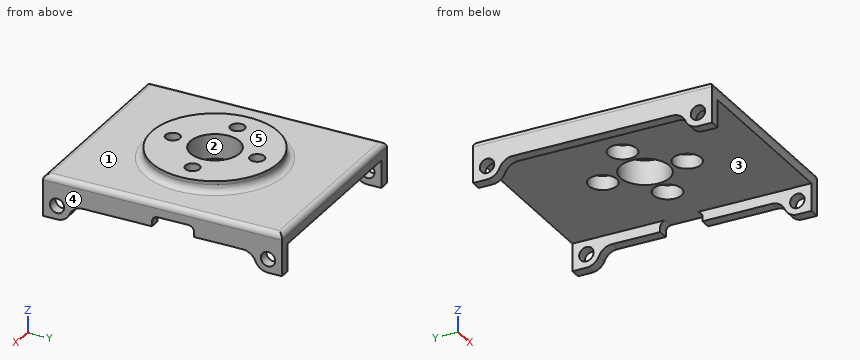
```python
from build123d import *

# Parameters (mm, degrees)
BOSS_EXTRUDE1_DEPTH = 17
SKETCH2_R           = 1.025
CUT_EXTRUDE1_DEPTH  = 50
CUT_EXTRUDE2_DEPTH  = 50
FILLET1_R           = 2
SKETCH8_W           = 1.5
SKETCH8_H           = 6
CUT_EXTRUDE5_DEPTH  = 10
SKETCH9_R           = 9
BOSS_EXTRUDE2_DEPTH = 1.5
SKETCH7_R           = 3.5
SKETCH7_R_2         = 1.025
CUT_EXTRUDE6_DEPTH  = 10
SKETCH10_R          = 2
CUT_EXTRUDE7_DEPTH  = 2
FILLET2_R           = 1
FILLET3_R           = 0.8
FILLET4_R           = 0.8


with BuildPart() as part:
    # Sketch1 → Boss-Extrude1 (new body, symmetric)
    with BuildSketch(Plane(origin=(0, 0, 0), x_dir=(1, 0, 0), z_dir=(0, 1, 0))):
        Polygon((-14, 0), (14, 0), (14, 5.93), (12.5, 5.93), (12.5, 2), (-12.5, 2), (-12.5, 5.93), (-14, 5.93), align=None)
    extrude(amount=BOSS_EXTRUDE1_DEPTH, both=True)

    # Sketch2 → Cut-Extrude1 (cut, symmetric)
    with BuildSketch(Plane(origin=(-12.5, 0, 0), x_dir=(0, 0, -1), z_dir=(1, 0, 0))):
        with Locations((4, 15)):
            Circle(SKETCH2_R)
        with Locations((4, -15)):
            Circle(SKETCH2_R)
    extrude(amount=CUT_EXTRUDE1_DEPTH, both=True, mode=Mode.SUBTRACT)

    # Sketch3 → Cut-Extrude2 (cut, symmetric)
    with BuildSketch(Plane(origin=(14, 0, 0), x_dir=(0, 0, -1), z_dir=(1, 0, 0))):
        with BuildLine():
            Line((3.5, -13.135891634), (3.5, 13.135891634))
            ThreePointArc((3.5, 13.135891634), (5.174712731, 13.468677043), (5.93, 15))
            Line((5.93, 15), (5.93, -15))
            ThreePointArc((5.93, -15), (5.174712731, -13.468677043), (3.5, -13.135891634))
        make_face()
    extrude(amount=CUT_EXTRUDE2_DEPTH, both=True, mode=Mode.SUBTRACT)

    # Fillet1
    fillet1_edges = [part.edges().sort_by_distance(p)[0] for p in [
        (13.25, 13.135891634, -3.5),
        (-13.25, 13.135891634, -3.5),
        (13.25, -13.135891634, -3.5),
        (-13.25, -13.135891634, -3.5),
    ]]
    fillet(fillet1_edges, radius=FILLET1_R)

    # Sketch8 → Cut-Extrude5 (cut)
    with BuildSketch(Plane(origin=(14, 0, 0), x_dir=(0, 0, -1), z_dir=(1, 0, 0))):
        with Locations((2.75, 1.5)):
            Rectangle(SKETCH8_W, SKETCH8_H)
    extrude(amount=-CUT_EXTRUDE5_DEPTH, mode=Mode.SUBTRACT)

    # Sketch9 → Boss-Extrude2 (add)
    with BuildSketch(Plane.XY):
        Circle(SKETCH9_R)
    extrude(amount=BOSS_EXTRUDE2_DEPTH)

    # Sketch7 → Cut-Extrude6 (cut)
    with BuildSketch(Plane.XY.offset(-2)):
        Circle(SKETCH7_R)
        with Locations((0, 6)):
            Circle(SKETCH7_R_2)
        with Locations((0, -6)):
            Circle(SKETCH7_R_2)
        with Locations((6, 0)):
            Circle(SKETCH7_R_2)
        with Locations((-6, 0)):
            Circle(SKETCH7_R_2)
    extrude(amount=CUT_EXTRUDE6_DEPTH, mode=Mode.SUBTRACT)

    # Sketch10 → Cut-Extrude7 (cut)
    with BuildSketch(Plane(origin=(0, 0, -2), x_dir=(-1, 0, 0), z_dir=(0, 0, -1))):
        with Locations((0, 6)):
            Circle(SKETCH10_R)
        with Locations((-6, 0)):
            Circle(SKETCH10_R)
        with Locations((0, -6)):
            Circle(SKETCH10_R)
        with Locations((6, 0)):
            Circle(SKETCH10_R)
    extrude(amount=-CUT_EXTRUDE7_DEPTH, mode=Mode.SUBTRACT)

    # Fillet2
    fillet2_edges = [part.edges().sort_by_distance(p)[0] for p in [
        (-9, 0, 0),
    ]]
    fillet(fillet2_edges, radius=FILLET2_R)

    # Fillet3
    fillet3_edges = [part.edges().sort_by_distance(p)[0] for p in [
        (14, 0, 0),
        (-14, 0, 0),
        (0, 17, 0),
        (0, -17, 0),
    ]]
    fillet(fillet3_edges, radius=FILLET3_R)

    # Fillet4
    fillet4_edges = [part.edges().sort_by_distance(p)[0] for p in [
        (13.25, -1.5, -2),
        (13.25, 4.5, -2),
    ]]
    fillet(fillet4_edges, radius=FILLET4_R)


solid = part.part
```
Geometry: final body of the model. Coordinates: model frame, mm. Face numbers are marked on the shaded views. A direction names the side the tool comes from. Round coordinates to 2 decimals unless told otherwise and drop trailing zeros. Order: outer loops, then holes, each group sorted by start corner. A loop starts at its lowest first (then second) coordinate and runs counter-clockwise, first axis right, second up. Notation, with made-up numbers: (21.5, -28.5) -> (65.5, -28.5) arc R10 cw to (65.5, -20.5) -> close; hole circle Ø9 at (24.5, 61). An arc over 180 degrees is marked (long way). Use CSV: the item, a comma, the result in double quotes. Start each with the question number.
1) Set-up query: the marked faces 1 and 2. Return all of +Z, -Z, +X, -X, +Y, -Y with unobstructed straight access to the full face (end or side cutting, diameter ignored); none if empty.
2) Section A-A (y = 0). State how many separate pieces and enclosed holes the cut face has, and give its area (3 significant figures).
3) Material intervals for line 1 along X through (y, z) = (10, -2.5); line 2 along Y through (x, z) = (0, -0.55); line 3 along Y through (x, z) = (13.75, -4) (3 decimals), sorted ascending. Write a range as from..to.
4) Draft query along X for the marked faces 3, 4 and 5. Return one class per face: +X half, -X half, draft (parallel to the pull), parting line (faces both ways), or undercut.
5) Section D-D (y = -12.5). Return the cut outline in (x, z).
6) Section B-B (z = 0.5). Return the cut outline in (x, y) (3 decimals), and give its area (3 significant figures).
7) Section C-C (x = 10.75). Return the cut outline in (y, z), and give its area (3 significant figures).
8) First-contact query: pin 1 Ø8 at (x, y) = (3.5, 1) entering from -Z; pin 2 Ø1.6 at (x, y) = (13, 7.5) entering from -Z; pin 3 Ø1.2 at (x, y) = (-1, -6) entering from -Z. Flat tips, straight axial feed; report the tip coordinate or a pass-through.
Returned:
1,face 1,"+Z"
1,face 2,"+Z, -Z"
2,separate pieces,"4"
2,enclosed holes,"0"
2,area,"38.8 mm²"
3,line 1,"x = -14..-12.5, 12.5..14"
3,line 2,"y = -16.96..-8, -4..-3.5, 3.5..4, 8..16.96"
3,line 3,"y = -17..-16.025, -13.975..-12.69, 12.69..13.975, 16.025..17"
4,face 3,"undercut"
4,face 4,"+X half"
4,face 5,"draft"
5,outline,"(-14, -3.85) -> (-12.5, -3.85) -> (-12.5, -2) -> (12.5, -2) -> (12.5, -3.85) -> (14, -3.85) -> (14, -0.8) arc R0.8 ccw to (13.2, 0) -> (-13.2, 0) arc R0.8 ccw to (-14, -0.8) -> close"
6,outline,"circle Ø18.268 at (0, 0); hole circle Ø2.05 at (-6, 0); hole circle Ø7 at (0, 0); hole circle Ø2.05 at (0, -6); hole circle Ø2.05 at (0, 6); hole circle Ø2.05 at (6, 0)"
6,area,"210 mm²"
7,outline,"(-17, -2) -> (17, -2) -> (17, -0.8) arc R0.8 ccw to (16.2, 0) -> (-16.2, 0) arc R0.8 ccw to (-17, -0.8) -> close"
7,area,"67.7 mm²"
8,pin 1,"stops at z = -2"
8,pin 2,"stops at z = -3.5"
8,pin 3,"stops at z = 0"
